Model file for the job. Use its own axes, mm. A direction names the side the tool comes from. Coordinates: 2 decimals unless noted, no trailing zeros. Write each loop counter-clockwise with the first axis right and the second up, starting at its lowest first coordinate (ties: lowest second). Pieces come first, ordered by that corner, then holes. Notation, with made-up numbers: (-39.75, 59.25) - (9.25, 59.25) arc R11 ccw to (9.25, 76.25) - close; hole circle Ø11 at (24.25, -28.5). An arc over 180 degrees is marked (long way). Put each result on its own line as item: value. Start each with the question number.
1. Which spindle directions (+Z, -Z, +X, -X, +Y, -Y) get a long thin tool onto all of the face, cutting with end or side? Do faces 1 (the face through (3, 0, 0)), 2 (the face through (7, 1, 0)), 3 (the face through (-8, -2, 0)). Say none if no direction does.
2. Saw through at B-B, the plane y = 2.5. Write the cut outline in (x, z).
3. Saw through at A-A, the plane z = 0. Write the cut outline in (x, y).
4. Saw through at D-D, the plane z = 1.95. Write the cut outline in (x, y), plus the area to 3 significant figures.
5. Saw through at C-C, the plane x = 0. Write the cut outline in (y, z), plus the area to 3 significant figures.
6. Pull direction Z, two halves, no side cores. Call faces 4 (the face through (-1.39, 2.46, 1.06)), 5 (the face through (-2, 1, -2.4)), 6 (the face through (-5, -4, 0)), 7 (the face through (-2, 1, 2.4)): released by +Z, released by -Z, zero draft, split by the parting line, or undercut.
7. Drill centre lines: L1, parallel to Z at x = 3.2, y = 2.5; L2, parallel to Y at x = 6.3, z = 0; L3, parallel to X at y = -8, z = 1.55. Where is each one in solid material? Low to high. Write a range as from..to.
8. Drop flat-ended pins along their axis: P1, Ø2, axis at y = -6.5, z = -1.5, coming from the +X side; P2, Ø6, axis at x = 2.5, y = -5, coming from the +Z side; P3, Ø0.9, axis at y = 2.5, z = 0, coming from the +X side. Give the stop position or say it passes through.
```python
from build123d import *

# Parameters (mm, degrees)
SKETCH_1_W          = 16
SKETCH_1_H          = 4.8
SKETCH_1_R          = 1.75
EXTRUDE_1_DEPTH     = 5
SKETCH_2_R          = 1.5
CUT_EXTRUDE_1_DEPTH = 3
SKETCH_3_R          = 0.55
CUT_EXTRUDE_2_DEPTH = 4
SKETCH_5_W          = 3
SKETCH_5_H          = 4.8
EXTRUDE_2_DEPTH     = 9
SKETCH_6_R          = 0.6
CUT_EXTRUDE_3_DEPTH = 15.0000001


with BuildPart() as part:
    # 草图1 → 凸台-拉伸1 (new body)
    with BuildSketch(Plane(origin=(0, 0, 0), x_dir=(1, 0, 0), z_dir=(0, 1, 0))):
        Rectangle(SKETCH_1_W, SKETCH_1_H)
        Circle(SKETCH_1_R, mode=Mode.SUBTRACT)
    extrude(amount=EXTRUDE_1_DEPTH)

    # 草图2 → 切除-拉伸1 (cut)
    with BuildSketch(Plane(origin=(8, 0, 0), x_dir=(0, 0, -1), z_dir=(1, 0, 0))):
        with Locations((0, 2.5)):
            Circle(SKETCH_2_R)
    extrude(amount=-CUT_EXTRUDE_1_DEPTH, mode=Mode.SUBTRACT)

    # 草图3 → 切除-拉伸2 (cut)
    with BuildSketch(Plane(origin=(5, 0, 0), x_dir=(0, 0, -1), z_dir=(1, 0, 0))):
        with Locations((0, 2.5)):
            Circle(SKETCH_3_R)
    extrude(amount=-CUT_EXTRUDE_2_DEPTH, mode=Mode.SUBTRACT)

    # 草图5 → 凸台-拉伸2 (add)
    with BuildSketch(Plane.XZ):
        with Locations((-6.5, 0)):
            Rectangle(SKETCH_5_W, SKETCH_5_H)
    extrude(amount=EXTRUDE_2_DEPTH)

    # 草图6 → 切除-拉伸3 (cut, through all)
    with BuildSketch(Plane.XZ.offset(9)):
        with Locations((-6.465889023, 0)):
            Circle(SKETCH_6_R)
    extrude(amount=-CUT_EXTRUDE_3_DEPTH, mode=Mode.SUBTRACT)


solid = part.part
```
Final values:
1. face 1: +Z, -Z, +X, -Y
1. face 2: +X
1. face 3: +Z, -Z, -X, +Y, -Y
2. outline: (-8, -2.4) - (8, -2.4) - (8, -1.5) - (5, -1.5) - (5, -0.55) - (1.66, -0.55) arc R1.75 cw (long way) to (1.66, 0.55) - (5, 0.55) - (5, 1.5) - (8, 1.5) - (8, 2.4) - (-8, 2.4) - close; hole circle Ø1.2 at (-6.47, 0)
3. outline: (-8, -9) - (-7.07, -9) - (-7.07, 5) - (-8, 5) - close; (-5.87, -9) - (-5, -9) - (-5, 0) - (-1.75, 0) - (-1.75, 5) - (-5.87, 5) - close; (1.75, 0) - (8, 0) - (8, 1) - (5, 1) - (5, 1.95) - (1.75, 1.95) - close; (1.75, 3.05) - (5, 3.05) - (5, 4) - (8, 4) - (8, 5) - (1.75, 5) - close
4. outline: (-8, -9) - (-5, -9) - (-5, 0) - (8, 0) - (8, 5) - (-8, 5) - close
4. area: 107 mm²
5. outline: (0, -2.4) - (5, -2.4) - (5, -1.75) - (0, -1.75) - close; (0, 1.75) - (5, 1.75) - (5, 2.4) - (0, 2.4) - close
5. area: 6.50 mm²
6. face 4: undercut
6. face 5: released by -Z
6. face 6: zero draft
6. face 7: released by +Z
7. L1: z = -2.4..-0.55, 0.55..2.4
7. L2: y = 0..1, 4..5
7. L3: x = -8..-5
8. P1: stops at x = -5
8. P2: passes through
8. P3: stops at x = -1.69
